Check sheet for the modelled part. Datum: model origin and axes. Units: mm. Round coordinates to 2 decimals unless told otherwise and drop trailing zeros. Loops run counter-clockwise (first coordinate to the right, second up) from the corner with the lowest first, then second, coordinate; pieces in that order, holes last. Notation, with made-up numbers: (25, 59.5) - (41, 59.5) arc R15 ccw to (41, 85.5) - close; hole circle Ø5 at (35, 67.25). An arc over 180 degrees is marked (long way). Put each result on its own line as item: value.
```python
from build123d import *

# Parameters (mm, degrees)
DURCHGANGSLOCH_F_R_M561_D           = 62
DURCHGANGSLOCH_F_R_M561_ON_FACE_2_D = 62
DURCHGANGSLOCH_F_R_M561_ON_FACE_3_D = 62
DURCHGANGSLOCH_F_R_M561_ON_FACE_4_D = 62
DURCHGANGSLOCH_F_R_M561_ON_FACE_5_D = 62
DURCHGANGSLOCH_F_R_M561_ON_FACE_6_D = 62
DURCHGANGSLOCH_F_R_M561_ON_FACE_7_D = 62


with BuildPart() as part:
    # Skizze2 → Rotation-D_nn1 (revolve)
    with BuildSketch(Plane.XY, mode=Mode.PRIVATE) as rotation_d_nn1_sk:
        with BuildLine():
            Line((900, 1200), (900, 1100))
            ThreePointArc((900, 1100), (874.831455224, 1002.871413764), (805.660377358, 930.188679245))
            ThreePointArc((805.660377358, 930.188679245), (418.949720044, 758.675979848), (0, 700))
            Line((0, 700), (0, 701))
            ThreePointArc((0, 701), (418.674998916, 759.637503795), (805.132075472, 931.037735849))
            ThreePointArc((805.132075472, 931.037735849), (873.957297948, 1003.357056695), (899, 1100))
            Line((899, 1100), (899, 1200))
            Line((899, 1200), (900, 1200))
        make_face()
    revolve(rotation_d_nn1_sk.sketch.rotate(Axis((0, 0, 0), (0, 1, 0)), 90), axis=Axis((0, 0, 0), (0, 1, 0)))  # turned: the seam where the file's is

    # Durchgangsloch f_r M561 (through all)
    with Locations(Plane(origin=(691.658204037, 891.573961556, -263.075899291), x_dir=(-0.887685936, -0.460449431, 0), z_dir=(0.453546363, -0.87437773, -0.172508786))):
        with Locations((0, 0)):
            Hole(DURCHGANGSLOCH_F_R_M561_D / 2)

    # Durchgangsloch f_r M561 on face 2 (through all)
    with Locations(Plane(origin=(477.38816392, 891.573961556, 565.420676089), x_dir=(0, -0.390389007, -0.92065), z_dir=(0.313040927, -0.874377797, 0.370767914))):
        with Locations((0, 0)):
            Hole(DURCHGANGSLOCH_F_R_M561_ON_FACE_2_D / 2)

    # Durchgangsloch f_r M561 on face 3 (through all)
    with Locations(Plane(origin=(740, 891.573961556, 0), x_dir=(-0.874377752, -0.485245862, 0), z_dir=(0.485245862, -0.874377752, 0))):
        with Locations((0, 0)):
            Hole(DURCHGANGSLOCH_F_R_M561_ON_FACE_3_D / 2)

    # Durchgangsloch f_r M561 on face 4 (through all)
    with Locations(Plane(origin=(441.411735182, 804.577527635, -336.423364295), x_dir=(-0.954951729, -0.296761176, 0), z_dir=(0.289449942, -0.931424814, -0.220604956))):
        with Locations((0, 0)):
            Hole(DURCHGANGSLOCH_F_R_M561_ON_FACE_4_D / 2)

    # Durchgangsloch f_r M561 on face 5 (through all)
    with Locations(Plane(origin=(555, 804.577527635, 0), x_dir=(-0.931424773, -0.363933911, 0), z_dir=(0.363933911, -0.931424773, 0))):
        with Locations((0, 0)):
            Hole(DURCHGANGSLOCH_F_R_M561_ON_FACE_5_D / 2)

    # Durchgangsloch f_r M561 on face 6 (through all)
    with Locations(Plane(origin=(696.216488153, 891.573961556, 250.764035747), x_dir=(-0.886444368, -0.462835158, 0), z_dir=(0.456535009, -0.874378016, 0.164435003))):
        with Locations((0, 0)):
            Hole(DURCHGANGSLOCH_F_R_M561_ON_FACE_6_D / 2)

    # Durchgangsloch f_r M561 on face 7 (through all)
    with Locations(Plane(origin=(451.200489776, 804.577527635, 323.176605011), x_dir=(-0.953071571, -0.302745076, 0), z_dir=(0.295868903, -0.931424693, 0.21191893))):
        with Locations((1e-09, 0)):
            Hole(DURCHGANGSLOCH_F_R_M561_ON_FACE_7_D / 2)


solid = part.part
```
Item 1: Section check C-C on y = 1071.5. Enter the section's corners in (x, z).
Filled sheet:
outline: circle Ø1795.92 at (0, 0); hole circle Ø1793.9 at (0, 0)
Item 2: Release check for a two-part mould opening along X. For faces 1 (the cylindrical face through (877.62, 1150.7, 194.89)), 2 (the cylindrical face through (468.8, 816.1, -345.3)), 3 (the cylindrical face through (-270.34, 1149.3, -858.44)) record: +X half, -X half, draft (parallel to the pull), parting line (faces both ways), or undercut.
Filled sheet:
face 1: undercut
face 2: undercut
face 3: parting line
Item 3: Section check B-B on x = 0. Enter the section's corners in (y, z), then the cut area to 3 significant figures.
Filled sheet:
outline: (930.19, -805.66) arc R200 ccw to (1100, -900) - (1200, -900) - (1200, -899) - (1100, -899) arc R199 cw to (931.04, -805.13) arc R1524 cw to (931.04, 805.13) arc R199 cw to (1100, 899) - (1200, 899) - (1200, 900) - (1100, 900) arc R200 ccw to (930.19, 805.66) arc R1525 ccw to start
area: 2,300 mm²
Item 4: Section check A-A on z = 0. Enter the section's corners in (x, y), then the cut area to 3 significant figures.
Filled sheet:
outline: (-900, 1100) arc R200 ccw to (-805.66, 930.19) arc R1525 ccw to (526.01, 793.59) - (525.65, 794.52) arc R1524 cw to (-805.13, 931.04) arc R199 cw to (-899, 1100) - (-899, 1200) - (-900, 1200) - close; (583.4, 817.08) - (583.76, 816.15) arc R1525 ccw to (712.74, 876.81) - (712.26, 877.68) arc R1524 cw to start; (766.47, 907.77) - (766.95, 906.89) arc R1525 ccw to (805.66, 930.19) arc R200 ccw to (900, 1100) - (900, 1200) - (899, 1200) - (899, 1100) arc R199 cw to (805.13, 931.04) arc R1524 cw to start
area: 2,180 mm²
Item 5: Thickness scan on line 1 (X direction, y = 1174, z = 0); line 2 (X direction, y = 868.5, z = 434); line 3 (Z direction, x = -426, y = 950.5). Record the ranges inside material, lowest first. Write a range as from..to.
Filled sheet:
line 1: -900..-899, 899..900
line 2: -545.14..-542.34, 542.34..545.14
line 3: -715.66..-713.9, 713.9..715.66
Item 6: Go/stop test with flat-tipped pins: pin 1 (6 mm diameter, centred on x = 292.5, z = -122, fed in from -Y); pin 2 (5 mm diameter, centred on x = -233.5, z = -464, fed in from -Y); pin 3 (12 mm diameter, centred on x = -241.5, z = 329, fed in from -Y). Record where each tip stops, or that it passes through.
Filled sheet:
pin 1: y = 732.66
pin 2: y = 790.29
pin 3: y = 753.97
